from build123d import *
from OCP.BRepFilletAPI import BRepFilletAPI_MakeChamfer

# Parameters (mm, degrees)
SKETCH1_R           = 15
BOSS_EXTRUDE1_DEPTH = 24.060856
SKETCH2_R           = 11.588546068
CUT_EXTRUDE1_DEPTH  = 33.076857568
CHAMFER1_SIZE       = 1.645344
CHAMFER1_SIZE2      = 0.94994


with BuildPart() as part:
    # Sketch1 → Boss-Extrude1 (new body)
    with BuildSketch(Plane(origin=(0, 0, 0), x_dir=(1, 0, 0), z_dir=(0, 1, 0))):
        with Locations(Location((0, 0, 0), (0, 0, 270))):
            Circle(SKETCH1_R)
    extrude(amount=BOSS_EXTRUDE1_DEPTH)

    # Sketch2 → Cut-Extrude1 (cut, through all)
    with BuildSketch(Plane(origin=(0, 0, 0), x_dir=(1, 0, 0), z_dir=(0, 1, 0))):
        with Locations(Location((0, 0, 0), (0, 0, 270))):
            Circle(SKETCH2_R)
    extrude(amount=CUT_EXTRUDE1_DEPTH, mode=Mode.SUBTRACT)

    # Chamfer1: one chamfer whose edges measure the first distance from different faces: ONE call of the kernel's chamfer builder (chamfer() names one face for all edges)
    chamfer1_edges_1 = [part.edges().sort_by_distance(p)[0] for p in [
        (0, 0, -15),
    ]]
    chamfer1_side_1 = [part.faces().sort_by_distance(p)[0] for p in [
        (0, 0, -14.575735931),
    ]]
    chamfer1_edges_2 = [part.edges().sort_by_distance(p)[0] for p in [
        (0, 24.060856, -15),
    ]]
    chamfer1_side_2 = [part.faces().sort_by_distance(p)[0] for p in [
        (0, 12.030428, -15),
    ]]
    chamfer1_edges_3 = [part.edges().sort_by_distance(p)[0] for p in [
        (0, 0, -11.588546068),
    ]]
    chamfer1_side_3 = [part.faces().sort_by_distance(p)[0] for p in [
        (0, 12.030428, -11.588546068),
    ]]
    chamfer1_edges_4 = [part.edges().sort_by_distance(p)[0] for p in [
        (0, 24.060856, -11.588546068),
    ]]
    chamfer1_side_4 = [part.faces().sort_by_distance(p)[0] for p in [
        (0, 24.060856, -14.575735931),
    ]]
    chamfer1 = BRepFilletAPI_MakeChamfer(part.part.solid().wrapped)
    for e in chamfer1_edges_1:
        chamfer1.Add(CHAMFER1_SIZE, CHAMFER1_SIZE2, e.wrapped, chamfer1_side_1[0].wrapped)  # the first distance lies on this face
    for e in chamfer1_edges_2:
        chamfer1.Add(CHAMFER1_SIZE, CHAMFER1_SIZE2, e.wrapped, chamfer1_side_2[0].wrapped)  # the first distance lies on this face
    for e in chamfer1_edges_3:
        chamfer1.Add(CHAMFER1_SIZE, CHAMFER1_SIZE2, e.wrapped, chamfer1_side_3[0].wrapped)  # the first distance lies on this face
    for e in chamfer1_edges_4:
        chamfer1.Add(CHAMFER1_SIZE, CHAMFER1_SIZE2, e.wrapped, chamfer1_side_4[0].wrapped)  # the first distance lies on this face
    add(Compound.cast(chamfer1.Shape()), mode=Mode.REPLACE)


solid = part.part
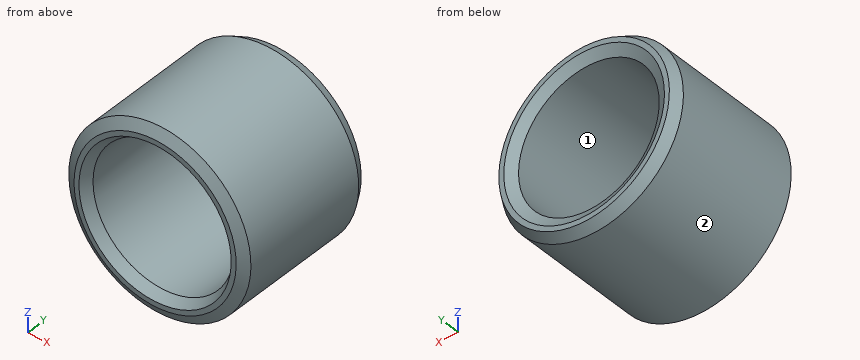
Check sheet for the modelled part. Datum: model origin and axes. Units: mm. Face numbers are marked on the shaded views. Give positions to 0.01 mm unless a question says otherwise; leave off trailing zeros. Write each loop counter-clockwise with the first axis right and the second up, starting at its lowest first coordinate (ties: lowest second). Pieces come first, ordered by that corner, then holes. Notation, with made-up numbers: (38, -34) -> (80, -34) arc R30 cw to (80, -5) -> close; hole circle Ø7 at (48.25, -27). An arc over 180 degrees is marked (long way). Use one line per item in the form item = value. Start each with the question number.
1. Section check A-A (x = 0). Record the cut outline in (y, z), and give its area (3 significant figures).
2. Section check B-B (z = 0). Record the cut outline in (x, y), and give its area (3 significant figures).
3. Go/stop test with flat-tipped pins: P1, Ø1.5, axis at x = 9, z = 1.5, coming from the -Y side; P2, Ø6, axis at x = -11.5, y = 9, coming from the -Z side; P3, Ø2, axis at y = 9, z = 3.5, coming from the -X side; P4, Ø6, axis at y = 19, z = -9, coming from the +X side. Record where each tip stops, or that it passes through.
4. Section check C-C (y = 21). Record the cut outline in (x, z), and give its area (3 significant figures).
5. Thickness scan on line 1 along X through (y, z) = (11, 0); line 2 along Z through (x, y) = (4.25, 5); line 3 along Z through (x, y) = (-6, 21). Record the ranges inside material, lowest first. Write a range as from..to.
6. Mould release check, pull along Z, two halves, no side actions. Record for the marked faces 1 and 2: pulls with the +Z half, pulls with the -Z half, needs draft (parallel to the pull), parting line crosses it, or undercut.
Conclusion:
q1.outline = (0, -13.35) -> (0.95, -15) -> (22.42, -15) -> (24.06, -14.05) -> (24.06, -13.23) -> (23.11, -11.59) -> (1.65, -11.59) -> (0, -12.54) -> close; (0, 12.54) -> (1.65, 11.59) -> (23.11, 11.59) -> (24.06, 13.23) -> (24.06, 14.05) -> (22.42, 15) -> (0.95, 15) -> (0, 13.35) -> close
q1.area = 158 mm²
q2.outline = (-15, 0.95) -> (-13.35, 0) -> (-12.54, 0) -> (-11.59, 1.65) -> (-11.59, 23.11) -> (-13.23, 24.06) -> (-14.05, 24.06) -> (-15, 22.42) -> close; (11.59, 1.65) -> (12.54, 0) -> (13.35, 0) -> (15, 0.95) -> (15, 22.42) -> (14.05, 24.06) -> (13.23, 24.06) -> (11.59, 23.11) -> close
q2.area = 158 mm²
q3.P1 = through
q3.P2 = -12.36
q3.P3 = -14.79
q3.P4 = 13.75
q4.outline = circle Ø30 at (0, 0); hole circle Ø23.18 at (0, 0)
q4.area = 285 mm²
q5.line_1 = -15..-11.59, 11.59..15
q5.line_2 = -14.39..-10.78, 10.78..14.39
q5.line_3 = -13.75..-9.91, 9.91..13.75
q6.face_1 = undercut
q6.face_2 = parting line crosses it
